Solid Edge part; units mm, degrees
sketch "Sketch1" plane through (0, 0, 0) normal (0, -1, 0) x (1, 0, 0)
  line L0 (0, 21.49) -> (6.51, 21.49)
  line L1 (6.51, 21.49) -> (6.51, 15.85)
  line L2 (6.51, 15.85) -> (3.6, 15.85)
  line L3 (3.6, 15.85) -> (3.6, 15.45)
  line L4 (3.6, 15.45) -> (4, 15.45)
  line L5 (4, 15.45) -> (4, 10.85)
  line L6 (4, 10.85) -> (3, 10.85)
  line L7 (3, 10.85) -> (3, 0)
  line L8 (3, 0) -> (0, 0)
  dimension "D1" = 6.51
  dimension "D2" = 3.6
  dimension "D3" = 3
  dimension "D4" = 4
  dimension "D5" = 3
revolve "RevolvedProtrusion1" add sketch "Sketch1" angle 360 about axis through (0, 0, 0) along (0, 0, 1)
chamfer "Chamfer1" distance 0.3 angle 45 3 edges at (-4, 0, 15.45) (-6.51, 0, 21.49) (-3, 0, 0)
fillet "Round_1" radius 0.2 4 edges at (-6.51, 0, 15.85) (-3.6, 0, 15.85) (-4, 0, 10.85) (-4, 0, 15.15)
sketch "Sketch2" plane through (0, 0, 21.49) normal (0, 0, 1) x (1, 0, 0)
  line L0 (2, 1.1547) -> (0, 2.3094)
  line L1 (0, 2.3094) -> (-2, 1.1547)
  line L2 (-2, 1.1547) -> (-2, -1.1547)
  line L3 (-2, -1.1547) -> (0, -2.3094)
  line L4 (0, -2.3094) -> (2, -1.1547)
  line L5 (2, -1.1547) -> (2, 1.1547)
extrude "ExtrudedCutout_1" cut sketch "Sketch2" against normal blind 3.3
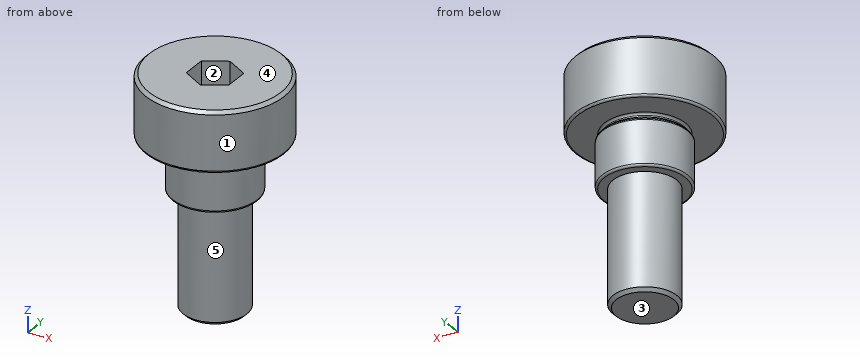
Model file for the job. Use its own axes, mm. Face numbers are marked on the shaded views. A direction names the side the tool comes from. Give positions to 0.01 mm unless a question says otherwise; leave off trailing zeros. Order: outer loops, then holes, each group sorted by start corner. A loop starts at its lowest first (then second) coordinate and runs counter-clockwise, first axis right, second up. Notation, with made-up numbers: (4.5, -35.5) - (22.5, -35.5) arc R16 ccw to (22.5, -7.5) - close; hole circle Ø2 at (73, -18). An arc over 180 degrees is marked (long way). One line per item, written item: value.
Item 1: Tool access for the marked faces 4 and 5: list every direction of +Z, -Z, +X, -X, +Y, -Y with a clear straight run to the whole face (end or side of a thin tool).
Response values:
face 4: +Z, +X, -X, +Y, -Y
face 5: -Z
Item 2: Pin check, flat tips, straight feed: pin 1 Ø4 at (y, z) = (-2, 10.5) entering from +X; pin 2 Ø1 at (x, y) = (-4, -4) entering from -Z; pin 3 Ø6 at (y, z) = (4.5, 16.5) entering from -X. Stop position of each tip, or through.
Response values:
pin 1: x = 4
pin 2: z = 15.85
pin 3: x = -6.33
Item 3: Slice it at C-C (z = 5). List the corners of the cut face in (x, y), then the cut area to 3 significant figures.
Response values:
outline: circle Ø6 at (0, 0)
area: 28.3 mm2
Item 4: Slice it at A-A (z = 19). List the corners of the cut face in (x, y), then the cut area to 3 significant figures.
Response values:
outline: circle Ø13.02 at (0, 0); hole (-2, -1.15) - (0, -2.31) - (2, -1.15) - (2, 1.15) - (0, 2.31) - (-2, 1.15) - close
area: 119 mm2
Item 5: Wall check: line 1 (Z direction, x = -1.5, y = 1.25); line 2 (X direction, y = -1.25, z = 18.25); line 3 (Z direction, x = 1.5, y = 5.25). Give the ranges that are in metal, low to high.
Response values:
line 1: 0 to 18.19
line 2: -6.39 to -1.83, 1.83 to 6.39
line 3: 15.85 to 21.49
Item 6: Slice it at B-B (z = 13.5). List the corners of the cut face in (x, y), then the cut area to 3 significant figures.
Response values:
outline: circle Ø8 at (0, 0)
area: 50.3 mm2
Item 7: Two-plate mould, pull along X, no slides. Class the marked faces 1, 2 and 3: released by +X, released by -X, zero draft, split by the parting line, or undercut.
Response values:
face 1: split by the parting line
face 2: undercut
face 3: zero draft
